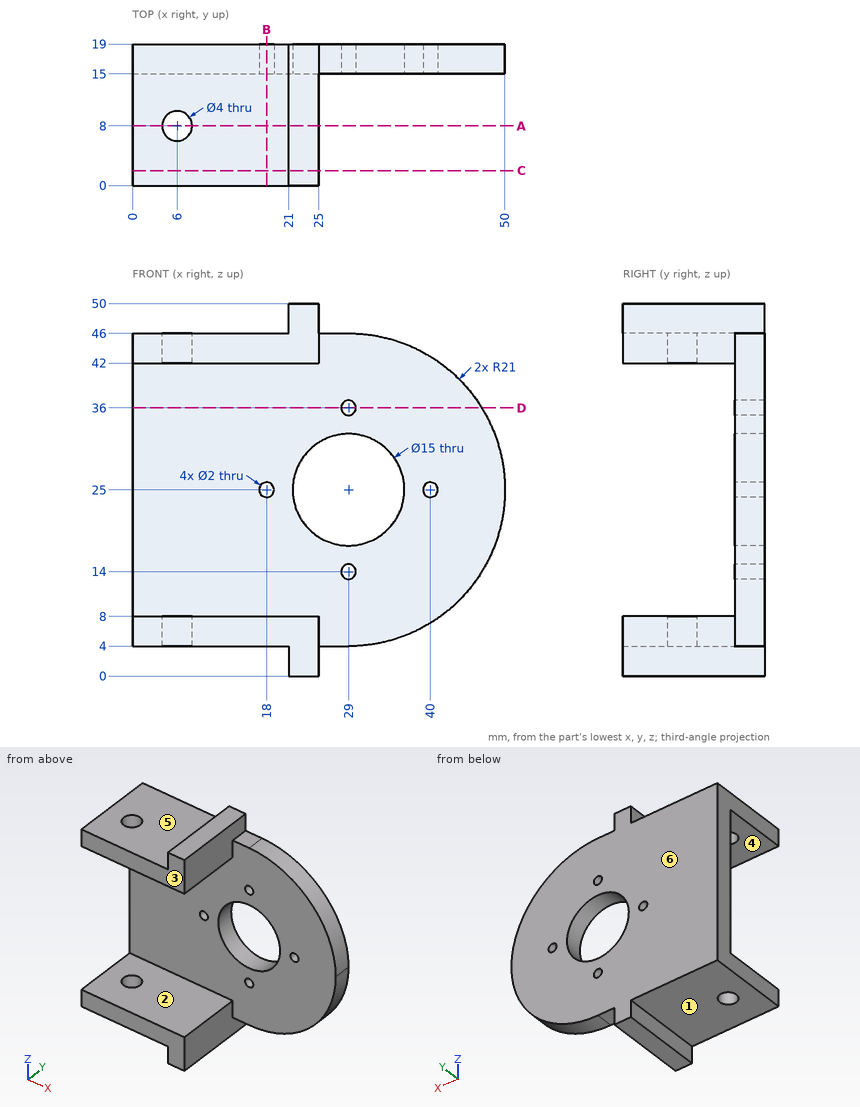
Can you work these out from the drawing? Everything is in mm from the part's minimum corner. A direction names the side the tool comes from. Give positions to 0.01 mm unless a question says otherwise; leave off trailing zeros. Write each loop counter-clockwise with the first axis right and the second up, starting at its lowest first coordinate (ties: lowest second). Pieces come first, ordered by that corner, then holes. Notation, with made-up numbers: (28, -6.5) -> (68, -6.5) arc R28 cw to (68, 26.5) -> close; hole circle Ø9 at (-33, 48.5). An arc over 180 degrees is marked (long way). Write each question's results on one line, items separated by ' | '. Start each with the question number.
Q1. I need wall thicknesses on probe 1 along Y at (x, z) = (6, 5.1); probe 2 along Z at (x, y) = (11, 2.5); probe 3 along X at (y, z) = (8, 43.7). Which ranges of each line are inside material? Lowest first, please.
Q2. Suppose I cut it at C-C, the plane y = 2. List the corners of the cut face in (x, z) for me, and give its area (3 significant figures).
Q3. Suppose I cut it at A-A, the plane y = 8. List the corners of the cut face in (x, z) for me.
Q4. Suppose I cut it at D-D, the plane z = 36. List the corners of the cut face in (x, y) for me.
Q5. Which directions (+Z, -Z, +X, -X, +Y, -Y) give clear straight access to the entire face, cutting with the end or side of a thin tool? Please do the marked faces 1, 2 and 3.
Q6. Suppose I cut it at B-B, the plane x = 18. List the corners of the cut face in (y, z) for me.
Q7. We'd pull the mould along Z, two halves only. Please class the marked faces 4, 5 and 6: +Z half, -Z half, draft (parallel to the pull), parting line (faces both ways), or undercut.
Q8. I'm going to push flat-ended pins straight in: pin 1 Ø2.5 at (y, z) = (7.5, 47) entering from +X; pin 2 Ø1.5 at (x, z) = (5, 24.5) entering from -Y; pin 3 Ø5 at (x, y) = (6, 8) entering from +Z. Where does each tip first touch, or does it pass through?
Outcome:
1) probe 1: 0 to 6, 10 to 19 | probe 2: 4 to 8, 42 to 46 | probe 3: 0 to 4, 8 to 25
2) outline: (0, 4) -> (21, 4) -> (21, 0) -> (25, 0) -> (25, 8) -> (0, 8) -> close; (0, 42) -> (25, 42) -> (25, 50) -> (21, 50) -> (21, 46) -> (0, 46) -> close | area: 232 mm2
3) outline: (0, 4) -> (4, 4) -> (4, 8) -> (0, 8) -> close; (0, 42) -> (4, 42) -> (4, 46) -> (0, 46) -> close; (8, 4) -> (21, 4) -> (21, 0) -> (25, 0) -> (25, 8) -> (8, 8) -> close; (8, 42) -> (25, 42) -> (25, 50) -> (21, 50) -> (21, 46) -> (8, 46) -> close
4) outline: (0, 15) -> (28, 15) -> (28, 19) -> (0, 19) -> close; (30, 15) -> (46.89, 15) -> (46.89, 19) -> (30, 19) -> close
5) face 1: -Z, -X, +Y, -Y | face 2: +X, -X, -Y | face 3: +Z, -Z, +X, -X, -Y
6) outline: (0, 4) -> (19, 4) -> (19, 24) -> (15, 24) -> (15, 8) -> (0, 8) -> close; (0, 42) -> (15, 42) -> (15, 26) -> (19, 26) -> (19, 46) -> (0, 46) -> close
7) face 4: undercut | face 5: +Z half | face 6: draft
8) pin 1: x = 25 | pin 2: y = 15 | pin 3: z = 46
